Design review of the part built by this model. Coordinates are the model's own, in mm. A direction names the side the tool comes from. Round coordinates to 2 decimals unless told otherwise and drop trailing zeros. Order: outer loops, then holes, each group sorted by start corner. A loop starts at its lowest first (then second) coordinate and runs counter-clockwise, first axis right, second up.
from build123d import *

# Parameters (mm, degrees)
SKETCH1_W                  = 60
SKETCH1_H                  = 60
SKETCH1_R                  = 16
BOSS_EXTRUDE1_DEPTH        = 8
SKETCH2_R                  = 3
BOSS_EXTRUDE2_DEPTH        = 2.5
SKETCH7_R                  = 3
BOSS_EXTRUDE3_DEPTH        = 5
BOSS_EXTRUDE4_DEPTH        = 5
BOSS_EXTRUDE5_START        = -1.4
SKETCH9_R                  = 16
SKETCH9_R_2                = 8
BOSS_EXTRUDE5_DEPTH        = 1.4
SKETCH10_R                 = 1.55
CUT_EXTRUDE2_DEPTH         = 44.17406629
CIRPATTERN1_COUNT          = 6
M3_TAPPED_HOLE2_AT_2_COUNT = 2
M3_TAPPED_HOLE2_AT_2_PITCH = 22
M3_TAPPED_HOLE2_AT_3_COUNT = 2
M3_TAPPED_HOLE2_AT_3_PITCH = 44


with BuildPart() as part:
    # Sketch1 → Boss-Extrude1 (new body)
    with BuildSketch(Plane(origin=(0, 0, 0), x_dir=(1, 0, 0), z_dir=(0, 1, 0))):
        Rectangle(SKETCH1_W, SKETCH1_H)
        with Locations(Location((0, 10, 0), (0, 0, 270))):
            Circle(SKETCH1_R, mode=Mode.SUBTRACT)
    extrude(amount=BOSS_EXTRUDE1_DEPTH)

    # Sketch2 → Boss-Extrude2 (add)
    with BuildSketch(Plane(origin=(0, 8, 0), x_dir=(1, 0, 0), z_dir=(0, 1, 0))):
        with Locations(Location((-17.5, -20.310889132, 0), (0, 0, 270))):
            Circle(SKETCH2_R)
        with Locations(Location((17.5, -20.310889132, 0), (0, 0, 270))):
            Circle(SKETCH2_R)
    extrude(amount=BOSS_EXTRUDE2_DEPTH)

    # Sketch7 → Boss-Extrude3 (add)
    with BuildSketch(Plane(origin=(0, 10.5, 0), x_dir=(1, 0, 0), z_dir=(0, 1, 0))):
        with Locations(Location((17.5, -20.310889132, 0), (0, 0, 270))):
            Circle(SKETCH7_R)
    extrude(amount=BOSS_EXTRUDE3_DEPTH)

    # Sketch8 → Boss-Extrude4 (add)
    with BuildSketch(Plane(origin=(0, 8, 0), x_dir=(1, 0, 0), z_dir=(0, 1, 0))):
        with BuildLine():
            ThreePointArc((13.339285714, -28.851290565), (27, -20.310889132), (13.339285714, -11.7704877))
            ThreePointArc((13.339285714, -11.7704877), (14.5, -20.310889132), (13.339285714, -28.851290565))
        make_face()
    extrude(amount=BOSS_EXTRUDE4_DEPTH)

    # Sketch9 → Boss-Extrude5 (add)
    with BuildSketch(Plane(origin=(0, 8, 0), x_dir=(1, 0, 0), z_dir=(0, 1, 0)).offset(BOSS_EXTRUDE5_START)):
        with Locations(Location((0, 10, 0), (0, 0, 270))):
            Circle(SKETCH9_R)
        with Locations(Location((0, 10, 0), (0, 0, 270))):
            Circle(SKETCH9_R_2, mode=Mode.SUBTRACT)
    extrude(amount=BOSS_EXTRUDE5_DEPTH)

    # Sketch10 → Cut-Extrude2 (cut, through all)
    with BuildSketch(Plane(origin=(0, 8, 0), x_dir=(1, 0, 0), z_dir=(0, 1, 0))):
        with Locations(Location((0, 21, 0), (0, 0, 270))):
            Circle(SKETCH10_R)
    cut_extrude2 = extrude(amount=-CUT_EXTRUDE2_DEPTH, mode=Mode.SUBTRACT)

    # CirPattern1: Cut-Extrude2 ×6 about axis
    cirpattern1_axis = Axis((0, 0, -10), (0, 1, 0))
    for i in range(1, CIRPATTERN1_COUNT):
        add(cut_extrude2.rotate(cirpattern1_axis, i * 360 / CIRPATTERN1_COUNT), mode=Mode.SUBTRACT)

    # Sketch16 → M3 Tapped Hole2 (revolve, cut)
    with BuildSketch(Plane(origin=(30, 4, 22), x_dir=(0, 0, -1), z_dir=(0, 1, 0))):
        Polygon((0, 0), (0, 8.251075774), (1.25, 7.5), (1.25, 0), align=None)
    m3_tapped_hole2 = revolve(axis=Axis((36.35, 4, 22), (-1, 0, 0)), mode=Mode.SUBTRACT)

    # M3 Tapped Hole2 at 2: M3 Tapped Hole2 ×2
    with Locations(*[(0, 0, -i * M3_TAPPED_HOLE2_AT_2_PITCH) for i in range(1, M3_TAPPED_HOLE2_AT_2_COUNT)]):
        add(m3_tapped_hole2, mode=Mode.SUBTRACT)

    # M3 Tapped Hole2 at 3: M3 Tapped Hole2 ×2
    with Locations(*[(0, 0, -i * M3_TAPPED_HOLE2_AT_3_PITCH) for i in range(1, M3_TAPPED_HOLE2_AT_3_COUNT)]):
        add(m3_tapped_hole2, mode=Mode.SUBTRACT)

    # Mirror1: M3 Tapped Hole2 across plane
    add(m3_tapped_hole2.mirror(Plane(origin=(0, 0, 0), x_dir=(0, 0, 1), z_dir=(1, 0, 0))), mode=Mode.SUBTRACT)

    # Mirror1 copy 1 sketch → Mirror1 copy 1 (revolve, cut)
    with BuildSketch(Plane(origin=(-30, 4, 0), x_dir=(0, 0, -1), z_dir=(0, 1, 0))):
        Polygon((0, 0), (0, -8.251075774), (1.25, -7.5), (1.25, 0), align=None)
    revolve(axis=Axis((-36.35, 4, 0), (-1, 0, 0)), mode=Mode.SUBTRACT)

    # Mirror1 copy 2 sketch → Mirror1 copy 2 (revolve, cut)
    with BuildSketch(Plane(origin=(-30, 4, -22), x_dir=(0, 0, -1), z_dir=(0, 1, 0))):
        Polygon((0, 0), (0, -8.251075774), (1.25, -7.5), (1.25, 0), align=None)
    revolve(axis=Axis((-36.35, 4, -22), (-1, 0, 0)), mode=Mode.SUBTRACT)


solid = part.part
1) Take a section at C-C on x = -17.5. Give the boundary of the cut face in (y, z), plus the area to 3 significant figures.
Results:
outline: (0, -30) - (8, -30) - (8, 17.31) - (10.5, 17.31) - (10.5, 23.31) - (8, 23.31) - (8, 30) - (0, 30) - close
area: 495 mm2
2) Take a section at A-A on x = 0. Give the boundary of the cut face in (y, z).
Results:
outline: (0, -30) - (8, -30) - (8, -22.55) - (6.6, -22.55) - (6.6, -26) - (0, -26) - close; (0, 6) - (6.6, 6) - (6.6, 2.55) - (8, 2.55) - (8, 30) - (0, 30) - close; (6.6, -19.45) - (8, -19.45) - (8, -18) - (6.6, -18) - close; (6.6, -2) - (8, -2) - (8, -0.55) - (6.6, -0.55) - close
3) Take a section at D-D on z = -24. Give the boundary of the cut face in (x, y), plus the area to 3 significant figures.
Results:
outline: (-30, 0) - (-7.75, 0) - (-7.75, 6.6) - (7.75, 6.6) - (7.75, 0) - (30, 0) - (30, 8) - (-30, 8) - close
area: 378 mm2
4) To check wall thickness, follow line 1 along Z through (x, y) = (28.75, 4); line 2 along X through (y, z) = (7.1, -15.5); line 3 along Y through (x, z) = (26, 0). State the ranges of each line that lie inside material, in increasing order.
Results:
line 1: z = -30 to -23.25, -20.75 to -1.25, 1.25 to 20.75, 23.25 to 30
line 2: x = -30 to -11.08, -7.98 to -5.81, 5.81 to 7.98, 11.08 to 30
line 3: y = 0 to 2.75, 5.25 to 8
5) The part is to be moulded in two halves that separate along X. For faces 1 (the face through (-21.88, 4.08, 21.8)), 2 (the face through (-9.736, 3.254, -22.697)), 3 (the face through (30, 2, 0)), 4 (the face through (-26.303, 4.479, -23.155)), say which applies: released by +X, released by -X, zero draft, split by the parting line, or undercut.
Results:
face 1: released by -X
face 2: undercut
face 3: released by +X
face 4: zero draft
6) Clearance check with flat-ended pins moving along their axes: P1, Ø5, axis at x = 0, z = -21, coming from the +Y side; P2, Ø4, axis at x = 23, z = 24, coming from the +Y side; P3, Ø4, axis at x = 9.53, z = -4.5, coming from the -Y side. State where each tip first meets the part, or that it passes through.
Results:
P1: stops at y = 8
P2: stops at y = 13
P3: stops at y = 6.6
7) Take a section at B-B on z = -10. Give the boundary of the cut face in (x, y).
Results:
outline: (-30, 0) - (-16, 0) - (-16, 6.6) - (-8, 6.6) - (-8, 8) - (-30, 8) - close; (8, 6.6) - (16, 6.6) - (16, 0) - (30, 0) - (30, 8) - (8, 8) - close
8) For faces 5 (the face through (-30, 2, 0)), 6 (the face through (26.996, 10.465, 20.58)), 7 (the face through (26.3, 5.22, 0.27)), 8 (the face through (-26.3, 5.22, 0.27)), list the 3-axis set-ups (+Z, -Z, +X, -X, +Y, -Y) from which the entire face can be reached by the end or side of a thin tool; tool diameter is ignored.
Results:
face 5: +Z, -Z, -X, +Y, -Y
face 6: +Y
face 7: +X
face 8: -X
